from build123d import *

# Parameters (mm, degrees)
SKETCH_1_R      = 20
SKETCH_1_R_2    = 7.5
EXTRUDE_1_DEPTH = 1.5
SKETCH_2_W      = 9.284271247
SKETCH_2_H      = 4
SKETCH_2_W_2    = 4
SKETCH_2_H_2    = 9.284271247
EXTRUDE_2_DEPTH = 1.5


with BuildPart() as part:
    # 草图1 → 凸台-拉伸1 (new body)
    with BuildSketch(Plane.XY):
        Circle(SKETCH_1_R)
        Circle(SKETCH_1_R_2, mode=Mode.SUBTRACT)
    extrude(amount=EXTRUDE_1_DEPTH)

    # 草图2 → 凸台-拉伸2 (add)
    with BuildSketch(Plane.XY):
        with Locations((23.642135624, 0)):
            Rectangle(SKETCH_2_W, SKETCH_2_H)
        with Locations((0, 23.642135624)):
            Rectangle(SKETCH_2_W_2, SKETCH_2_H_2)
        with Locations((-23.642135624, 0)):
            Rectangle(SKETCH_2_W, SKETCH_2_H)
        with Locations((0, -23.642135624)):
            Rectangle(SKETCH_2_W_2, SKETCH_2_H_2)
    extrude(amount=EXTRUDE_2_DEPTH)


solid = part.part
Could you check a few things on this model? Use its own coordinates, in mm. A direction names the side the tool comes from. Round coordinates to 2 decimals unless told otherwise and drop trailing zeros. Order: outer loops, then holes, each group sorted by start corner. A loop starts at its lowest first (then second) coordinate and runs counter-clockwise, first axis right, second up.
(1) Imagine slicing it at D-D (y = -24.5). Write out the boundary of the cut face in (x, z).
Response values:
outline: (-2, 0) - (2, 0) - (2, 1.5) - (-2, 1.5) - close
(2) If we mould it in two halves opening along X, with no side actions, what happens to faces 6 (the cylindrical face through (-7.493, 0.33, 0.74)), 7 (the flat face through (0, 28.284, 1)), 8 (the cylindrical face through (-14.006, 14.277, 0.74))? For each: released by +X, released by -X, zero draft, split by the parting line, or undercut.
Response values:
face 6: undercut
face 7: zero draft
face 8: released by -X
(3) Imagine slicing it at C-C (z = 0.8). Write out the boundary of the cut face in (x, y), plus the area to 3 significant figures.
Response values:
outline: (-28.28, -2) - (-19.9, -2) arc R20 ccw to (-2, -19.9) - (-2, -28.28) - (2, -28.28) - (2, -19.9) arc R20 ccw to (19.9, -2) - (28.28, -2) - (28.28, 2) - (19.9, 2) arc R20 ccw to (2, 19.9) - (2, 28.28) - (-2, 28.28) - (-2, 19.9) arc R20 ccw to (-19.9, 2) - (-28.28, 2) - close; hole circle Ø15 at (0, 0)
area: 1,210 mm2
(4) Which directions (+Z, -Z, +X, -X, +Y, -Y) give clear straight access to the entire face, cutting with the end or side of a thin tool? Please do faces 1 (the flat face through (2, 24, 1)), 2 (the flat face through (6, -6, 0)), 3 (the flat face through (-24, -2, 1)), 4 (the flat face through (2, -24, 1)), 5 (the flat face through (-2, 24, 1)).
Response values:
face 1: +Z, -Z, +X, +Y
face 2: -Z, +X, -X, +Y, -Y
face 3: +Z, -Z, -X, -Y
face 4: +Z, -Z, +X, -Y
face 5: +Z, -Z, -X, +Y
(5) Imagine slicing it at A-A (y = 0). Write out the boundary of the cut face in (x, z).
Response values:
outline: (-28.28, 0) - (-7.5, 0) - (-7.5, 1.5) - (-28.28, 1.5) - close; (7.5, 0) - (28.28, 0) - (28.28, 1.5) - (7.5, 1.5) - close
(6) Please list where these lines run through material, in increasing order: line 1 along Y through (x, z) = (0, 1); line 2 along X through (y, z) = (-24, 1.25); line 3 along Y through (x, z) = (-2.5, 0.4).
Response values:
line 1: y = -28.28 to -7.5, 7.5 to 28.28
line 2: x = -2 to 2
line 3: y = -19.84 to -7.07, 7.07 to 19.84
